Source: CAD feature listing. Evaluate the final solid. Frame: model axes, mm. A direction names the side the tool comes from. Coordinates: 2 decimals unless noted, no trailing zeros. Write each loop counter-clockwise with the first axis right and the second up, starting at its lowest first coordinate (ties: lowest second). Pieces come first, ordered by that corner, then holes. Notation, with made-up numbers: (-20.75, 81) - (13.25, 81) arc R28 cw to (13.25, 116) - close; hole circle Ø11 at (88, 61.25). An arc over 180 degrees is marked (long way). One line per item, written item: value.
from build123d import *

# Parameters (mm, degrees)
BOSS_EXTRUDE1_DEPTH = 6.9
CUT_EXTRUDE1_DEPTH  = 41.174882094
CUT_EXTRUDE2_DEPTH  = 41.174882094
HOLE1_D             = 3.4
HOLE2_D             = 3
HOLE2_CBORE_D       = 4.4
HOLE2_CBORE_DEPTH   = 2.8
FILLET1_R           = 0.6
FILLET2_R           = 5
CHAMFER2_SIZE       = 0.5


with BuildPart() as part:
    # Sketch1 → Boss-Extrude1 (new body)
    with BuildSketch(Plane(origin=(-30.446370889, 0, 0), x_dir=(0, 0, -1), z_dir=(1, 0, 0))):
        with BuildLine():
            Line((93.90701583, -40.982811072), (88.40701583, -52.223840783))
            ThreePointArc((88.40701583, -52.223840783), (90.242028227, -57.574796726), (95.59298417, -55.739784329))
            Line((95.59298417, -55.739784329), (101.09298417, -44.498754618))
            ThreePointArc((101.09298417, -44.498754618), (99.257971773, -39.147798675), (93.90701583, -40.982811072))
        make_face()
    extrude(amount=-BOSS_EXTRUDE1_DEPTH)

    # Sketch2 → Cut-Extrude1 (cut, through all)
    with BuildSketch(Plane(origin=(0, -48.50387467, -99.133362956), x_dir=(-1, 0, 0), z_dir=(0, -0.43949294330941685, -0.8982460424523036))):
        Polygon((37.346370889, 0.458822931), (33.846370889, -4.055598708), (33.846370889, -14.237691346), (37.346370889, -14.237691346), align=None)
    extrude(amount=-CUT_EXTRUDE1_DEPTH, mode=Mode.SUBTRACT)

    # Sketch3 → Cut-Extrude2 (cut, through all)
    with BuildSketch(Plane(origin=(0, -48.50387467, -99.133362956), x_dir=(-1, 0, 0), z_dir=(0, -0.4394929433094169, -0.8982460424523037))):
        with BuildLine():
            Line((29.844897196, 8.580951501), (29.844897196, -5.213665722))
            ThreePointArc((29.844897196, -5.213665722), (30.303827303, -3.12113514), (31.596370889, -1.412734673))
            Line((31.596370889, -1.412734673), (31.596370889, 8.580951501))
            Line((31.596370889, 8.580951501), (29.844897196, 8.580951501))
        make_face()
    extrude(amount=-CUT_EXTRUDE2_DEPTH, mode=Mode.SUBTRACT)

    # Hole1 (through all)
    with Locations(Plane(origin=(-30.446370889, 0, 0), x_dir=(0, 0, -1), z_dir=(1, 0, 0))):
        with Locations((92, -53.981812556)):
            Hole(HOLE1_D / 2)

    # Hole2 (through all)
    with Locations(Plane(origin=(-31.596370889, 0, 0), x_dir=(0, 0, -1), z_dir=(1, 0, 0))):
        with Locations((97.5, -42.740782845)):
            CounterBoreHole(HOLE2_D / 2, HOLE2_CBORE_D / 2, HOLE2_CBORE_DEPTH)

    # Fillet1
    fillet1_edges = [part.edges().sort_by_distance(p)[0] for p in [
        (-33.846370889, -50.388828386, -93.757971773),
        (-31.596370889, -48.014886226, -94.919491867),
    ]]
    fillet(fillet1_edges, radius=FILLET1_R)

    # Fillet2
    fillet2_edges = [part.edges().sort_by_distance(p)[0] for p in [
        (-37.346370889, -46.333767015, -95.742028227),
    ]]
    fillet(fillet2_edges, radius=FILLET2_R)

    # Chamfer2
    chamfer2_edges = [part.edges().sort_by_distance(p)[0] for p in [
        (-31.596370889, -42.740782845, -95.3),
    ]]
    chamfer(chamfer2_edges, length=CHAMFER2_SIZE)


solid = part.part
1) Contact query for flat-ended pins moving along their axis: P1, Ø1, axis at x = -32, y = -41, coming from the -Z side; P2, Ø6, axis at y = -49.5, z = -96, coming from the -X side; P3, Ø1, axis at x = -31.5, y = -51.5, coming from the -Z side. Output: stop coordinate, or through.
Values found:
P1: z = -101.3
P2: x = -37.13
P3: z = -97.91
2) Section query A-A on y = -53.25. Output: boundary loops of the cut face in (x, z), then the cut area to 3 significant figures.
Values found:
outline: (-33.85, -96.81) - (-30.45, -96.81) - (-30.45, -93.53) - (-33.85, -93.53) - close; (-33.85, -90.47) - (-30.45, -90.47) - (-30.45, -88.07) - (-33.85, -88.07) - close
area: 19.3 mm2
3) Reachability of faces 4 (the flat face through (-37.346, -42, -99)), 5 (the flat face through (-34.396, -42, -99)), 6 (the flat face through (-31.596, -45.5, -96.2)) from +Z, -Z, +X, -X, +Y, -Y: full face, straight path, thin tool, end or side. Return the list, or none.
Values found:
face 4: +Z, -Z, -X, +Y, -Y
face 5: +X
face 6: -Z, +X, +Y
4) Draft query along Z for faces 1 (the flat face through (-33.846, -52, -92)), 2 (the flat face through (-33.848, -48.949, -98.916)), 3 (the cylindrical face through (-33.23, -44.888, -97.023)). Return one class per face: released by +Z, released by -Z, zero draft, split by the parting line, or undercut.
Values found:
face 1: zero draft
face 2: released by -Z
face 3: undercut
5) Section query D-D on y = -39.75. Output: boundary loops of the cut face in (x, z), then the cut area to 3 significant figures.
Values found:
outline: (-37.35, -100.16) - (-31.6, -100.16) - (-31.6, -94.84) - (-37.35, -94.84) - close
area: 30.5 mm2
6) Material intervals for line 1 (X direction, y = -54, z = -95.75); line 2 (Y direction, x = -32.65, z = -92); line 3 (Y direction, x = -32, z = -95.5), sorted ascending.
Values found:
line 1: -33.85 to -30.45
line 2: -57.98 to -55.68, -52.28 to -44.88
line 3: -55.92 to -43.87, -41.61 to -39.28
